```python
from build123d import *

# Parameters (mm, degrees)
SKETCH1_W             = 245.11
SKETCH1_H             = 93.653112922
BOSS_EXTRUDE1_DEPTH   = 2.8575
CUT_EXTRUDE1_REACH    = 4.857
SKETCH2_W             = 181.61
SKETCH2_H             = 3.399764473
CUT_EXTRUDE3_REACH    = 4.857
SKETCH4_W             = 4.572
SKETCH4_H             = 11.676791988
SKETCH4_H_2           = 25.4
CHAMFER2_SIZE         = 0.762
CHAMFER2_SIZE2        = 1.319822715
CHAMFER2_PART_2_SIZE  = 0.762
CHAMFER2_PART_2_SIZE2 = 1.319822715
CHAMFER2_PART_3_SIZE  = 0.762
CHAMFER2_PART_3_SIZE2 = 1.319822715
CHAMFER3_SIZE         = 0.762
CHAMFER3_SIZE2        = 1.319822715
CHAMFER3_PART_2_SIZE  = 0.762
CHAMFER3_PART_2_SIZE2 = 1.319822715
CHAMFER3_PART_3_SIZE  = 0.762
CHAMFER3_PART_3_SIZE2 = 1.319822715
SKETCH6_W             = 11.684
SKETCH6_H             = 0.762
CUT_EXTRUDE4_DEPTH    = 3.8575
SKETCH9_W             = 2.86258
SKETCH9_H             = 12.192
CUT_EXTRUDE5_DEPTH    = 3.8575
SKETCH11_R            = 2.975
CUT_EXTRUDE6_DEPTH    = 3.8575


with BuildPart() as part:
    # Sketch1 → Boss-Extrude1 (new body)
    with BuildSketch(Plane(origin=(0, 0, 0), x_dir=(1, 0, 0), z_dir=(0, 1, 0))):
        Rectangle(SKETCH1_W, SKETCH1_H)
    extrude(amount=BOSS_EXTRUDE1_DEPTH)

    # Sketch2 → Cut-Extrude1 (cut, up to next)
    with BuildSketch(Plane(origin=(0, 2.8575, 0), x_dir=(1, 0, 0), z_dir=(0, 1, 0)), mode=Mode.PRIVATE) as cut_extrude1_sk1:
        with Locations((31.75, 45.126674225)):
            Rectangle(SKETCH2_W, SKETCH2_H)
    cut_extrude1_tool1 = extrude(cut_extrude1_sk1.sketch, amount=-CUT_EXTRUDE1_REACH, mode=Mode.PRIVATE) & part.part
    add(cut_extrude1_tool1.solids().sort_by_distance((31.75, 2.8575, -45.126674))[0], mode=Mode.SUBTRACT)
    # Sketch2 → Cut-Extrude1 (cut, up to next)
    with BuildSketch(Plane(origin=(0, 2.8575, 0), x_dir=(1, 0, 0), z_dir=(0, 1, 0)), mode=Mode.PRIVATE) as cut_extrude1_sk2:
        with Locations((31.75, -45.126674225)):
            Rectangle(SKETCH2_W, SKETCH2_H)
    cut_extrude1_tool2 = extrude(cut_extrude1_sk2.sketch, amount=-CUT_EXTRUDE1_REACH, mode=Mode.PRIVATE) & part.part
    add(cut_extrude1_tool2.solids().sort_by_distance((31.75, 2.8575, 45.126674))[0], mode=Mode.SUBTRACT)

    # Sketch4 → Cut-Extrude3 (cut, up to next)
    with BuildSketch(Plane(origin=(0, 2.8575, 0), x_dir=(1, 0, 0), z_dir=(0, 1, 0)), mode=Mode.PRIVATE) as cut_extrude3_sk1:
        with Locations((120.269, 37.588395994)):
            Rectangle(SKETCH4_W, SKETCH4_H)
    cut_extrude3_tool1 = extrude(cut_extrude3_sk1.sketch, amount=-CUT_EXTRUDE3_REACH, mode=Mode.PRIVATE) & part.part
    add(cut_extrude3_tool1.solids().sort_by_distance((120.269, 2.8575, -37.588396))[0], mode=Mode.SUBTRACT)
    # Sketch4 → Cut-Extrude3 (cut, up to next)
    with BuildSketch(Plane(origin=(0, 2.8575, 0), x_dir=(1, 0, 0), z_dir=(0, 1, 0)), mode=Mode.PRIVATE) as cut_extrude3_sk2:
        with Locations((120.269, -37.588395994)):
            Rectangle(SKETCH4_W, SKETCH4_H)
    cut_extrude3_tool2 = extrude(cut_extrude3_sk2.sketch, amount=-CUT_EXTRUDE3_REACH, mode=Mode.PRIVATE) & part.part
    add(cut_extrude3_tool2.solids().sort_by_distance((120.269, 2.8575, 37.588396))[0], mode=Mode.SUBTRACT)
    # Sketch4 → Cut-Extrude3 (cut, up to next)
    with BuildSketch(Plane(origin=(0, 2.8575, 0), x_dir=(1, 0, 0), z_dir=(0, 1, 0)), mode=Mode.PRIVATE) as cut_extrude3_sk3:
        with Locations((120.269, 0)):
            Rectangle(SKETCH4_W, SKETCH4_H_2)
    cut_extrude3_tool3 = extrude(cut_extrude3_sk3.sketch, amount=-CUT_EXTRUDE3_REACH, mode=Mode.PRIVATE) & part.part
    add(cut_extrude3_tool3.solids().sort_by_distance((120.269, 2.8575, 0))[0], mode=Mode.SUBTRACT)

    # Chamfer2
    chamfer2_edges = [part.edges().sort_by_distance(p)[0] for p in [
        (122.555, 1.42875, 31.75),
    ]]
    chamfer2_side = [part.faces().sort_by_distance(p)[0] for p in [
        (122.555, 1.42875, 22.225),
    ]]
    chamfer(chamfer2_edges, length=CHAMFER2_SIZE, length2=CHAMFER2_SIZE2, reference=chamfer2_side[0])

    # Chamfer2 part 2
    chamfer2_part_2_edges = [part.edges().sort_by_distance(p)[0] for p in [
        (117.983, 1.42875, 43.426791988),
    ]]
    chamfer2_part_2_side = [part.faces().sort_by_distance(p)[0] for p in [
        (117.983, 1.42875, 37.588395994),
    ]]
    chamfer(chamfer2_part_2_edges, length=CHAMFER2_PART_2_SIZE, length2=CHAMFER2_PART_2_SIZE2, reference=chamfer2_part_2_side[0])

    # Chamfer2 part 3
    chamfer2_part_3_edges = [part.edges().sort_by_distance(p)[0] for p in [
        (122.555, 1.42875, -12.7),
    ]]
    chamfer2_part_3_side = [part.faces().sort_by_distance(p)[0] for p in [
        (122.555, 1.42875, -22.225),
    ]]
    chamfer(chamfer2_part_3_edges, length=CHAMFER2_PART_3_SIZE, length2=CHAMFER2_PART_3_SIZE2, reference=chamfer2_part_3_side[0])

    # Chamfer3
    chamfer3_edges = [part.edges().sort_by_distance(p)[0] for p in [
        (122.555, 1.42875, -31.75),
    ]]
    chamfer3_side = [part.faces().sort_by_distance(p)[0] for p in [
        (122.555, 1.42875, -22.606),
    ]]
    chamfer(chamfer3_edges, length=CHAMFER3_SIZE, length2=CHAMFER3_SIZE2, reference=chamfer3_side[0])

    # Chamfer3 part 2
    chamfer3_part_2_edges = [part.edges().sort_by_distance(p)[0] for p in [
        (117.983, 1.42875, -43.426791988),
    ]]
    chamfer3_part_2_side = [part.faces().sort_by_distance(p)[0] for p in [
        (117.983, 1.42875, -37.588395994),
    ]]
    chamfer(chamfer3_part_2_edges, length=CHAMFER3_PART_2_SIZE, length2=CHAMFER3_PART_2_SIZE2, reference=chamfer3_part_2_side[0])

    # Chamfer3 part 3
    chamfer3_part_3_edges = [part.edges().sort_by_distance(p)[0] for p in [
        (122.555, 1.42875, 12.7),
    ]]
    chamfer3_part_3_side = [part.faces().sort_by_distance(p)[0] for p in [
        (122.555, 1.42875, 21.844),
    ]]
    chamfer(chamfer3_part_3_edges, length=CHAMFER3_PART_3_SIZE, length2=CHAMFER3_PART_3_SIZE2, reference=chamfer3_part_3_side[0])

    # Sketch6 → Cut-Extrude4 (cut, through all)
    with BuildSketch(Plane(origin=(0, 2.8575, 0), x_dir=(1, 0, 0), z_dir=(0, 1, 0))):
        with Locations((99.533234068, -0.475391988)):
            Rectangle(SKETCH6_W, SKETCH6_H)
        with Locations((99.533234068, -6.571391988)):
            Rectangle(SKETCH6_W, SKETCH6_H)
        with Locations((99.533234068, -17.802329902)):
            Rectangle(SKETCH6_W, SKETCH6_H)
        with Locations((99.533234068, -23.898329902)):
            Rectangle(SKETCH6_W, SKETCH6_H)
        with Locations((59.401234068, -0.475391988)):
            Rectangle(SKETCH6_W, SKETCH6_H)
        with Locations((59.401234068, -6.571391988)):
            Rectangle(SKETCH6_W, SKETCH6_H)
        with Locations((59.401234068, -17.802329902)):
            Rectangle(SKETCH6_W, SKETCH6_H)
        with Locations((59.401234068, -23.898329902)):
            Rectangle(SKETCH6_W, SKETCH6_H)
        with Locations((19.269234068, -0.475391988)):
            Rectangle(SKETCH6_W, SKETCH6_H)
        with Locations((19.269234068, -6.571391988)):
            Rectangle(SKETCH6_W, SKETCH6_H)
        with Locations((19.269234068, -17.802329902)):
            Rectangle(SKETCH6_W, SKETCH6_H)
        with Locations((19.269234068, -23.898329902)):
            Rectangle(SKETCH6_W, SKETCH6_H)
        with Locations((-20.862765932, -0.475391988)):
            Rectangle(SKETCH6_W, SKETCH6_H)
        with Locations((-20.862765932, -6.571391988)):
            Rectangle(SKETCH6_W, SKETCH6_H)
        with Locations((-20.862765932, -17.802329902)):
            Rectangle(SKETCH6_W, SKETCH6_H)
        with Locations((-20.862765932, -23.898329902)):
            Rectangle(SKETCH6_W, SKETCH6_H)
        with Locations((-60.994765932, -0.475391988)):
            Rectangle(SKETCH6_W, SKETCH6_H)
        with Locations((-60.994765932, -6.571391988)):
            Rectangle(SKETCH6_W, SKETCH6_H)
        with Locations((-60.994765932, -17.802329902)):
            Rectangle(SKETCH6_W, SKETCH6_H)
        with Locations((-60.994765932, -23.898329902)):
            Rectangle(SKETCH6_W, SKETCH6_H)
        with Locations((-101.126765932, -0.475391988)):
            Rectangle(SKETCH6_W, SKETCH6_H)
        with Locations((-101.126765932, -6.571391988)):
            Rectangle(SKETCH6_W, SKETCH6_H)
        with Locations((-101.126765932, -17.802329902)):
            Rectangle(SKETCH6_W, SKETCH6_H)
        with Locations((-101.126765932, -23.898329902)):
            Rectangle(SKETCH6_W, SKETCH6_H)
    extrude(amount=-CUT_EXTRUDE4_DEPTH, mode=Mode.SUBTRACT)

    # Sketch9 → Cut-Extrude5 (cut, through all)
    with BuildSketch(Plane(origin=(0, 2.8575, 0), x_dir=(1, 0, 0), z_dir=(0, 1, 0))):
        with Locations((80.97711923, 0.007208012)):
            Rectangle(SKETCH9_W, SKETCH9_H)
        with Locations((40.84511923, 0.007208012)):
            Rectangle(SKETCH9_W, SKETCH9_H)
        with Locations((40.84511923, -24.376791988)):
            Rectangle(SKETCH9_W, SKETCH9_H)
        with Locations((0.71311923, 0.007208012)):
            Rectangle(SKETCH9_W, SKETCH9_H)
        with Locations((0.71311923, -24.376791988)):
            Rectangle(SKETCH9_W, SKETCH9_H)
        with Locations((80.97711923, -24.376791988)):
            Rectangle(SKETCH9_W, SKETCH9_H)
        with Locations((-39.41888077, 0.007208012)):
            Rectangle(SKETCH9_W, SKETCH9_H)
        with Locations((-39.41888077, -24.376791988)):
            Rectangle(SKETCH9_W, SKETCH9_H)
        with Locations((-79.55088077, 0.007208012)):
            Rectangle(SKETCH9_W, SKETCH9_H)
        with Locations((-79.55088077, -24.376791988)):
            Rectangle(SKETCH9_W, SKETCH9_H)
    extrude(amount=-CUT_EXTRUDE5_DEPTH, mode=Mode.SUBTRACT)

    # Sketch11 → Cut-Extrude6 (cut, through all)
    with BuildSketch(Plane(origin=(0, 2.8575, 0), x_dir=(1, 0, 0), z_dir=(0, 1, 0))):
        with Locations((99.533234068, 13.215208012)):
            Circle(SKETCH11_R)
        with Locations((99.533234068, -37.584791988)):
            Circle(SKETCH11_R)
        with Locations((59.401234068, -37.584791988)):
            Circle(SKETCH11_R)
        with Locations((59.401234068, 13.215208012)):
            Circle(SKETCH11_R)
        with Locations((19.269234068, -37.584791988)):
            Circle(SKETCH11_R)
        with Locations((19.269234068, 13.215208012)):
            Circle(SKETCH11_R)
        with Locations((-20.862765932, -37.584791988)):
            Circle(SKETCH11_R)
        with Locations((-20.862765932, 13.215208012)):
            Circle(SKETCH11_R)
        with Locations((-60.994765932, -37.584791988)):
            Circle(SKETCH11_R)
        with Locations((-60.994765932, 13.215208012)):
            Circle(SKETCH11_R)
        with Locations((-101.126765932, -37.584791988)):
            Circle(SKETCH11_R)
        with Locations((-101.126765932, 13.215208012)):
            Circle(SKETCH11_R)
    extrude(amount=-CUT_EXTRUDE6_DEPTH, mode=Mode.SUBTRACT)


solid = part.part
```
Source: CAD feature listing. Evaluate the final solid. Frame: model axes, mm. Round coordinates to 2 decimals unless told otherwise and drop trailing zeros. Loops run counter-clockwise (first coordinate to the right, second up) from the corner with the lowest first, then second, coordinate; pieces in that order, holes last. Notation, with made-up numbers: M 6,46.25 L 27,46.25 A20 ccw 27,51.25 Z; hole C -6.5,-8.75 d3. An arc over 180 degrees is marked long. Use a Markdown table: item, result. Add a question column.
1. Cut plane C-C, the plane y = 1.1. State how many separate pieces and enclosed holes the cut face has, and give its area (3 significant figures).
2. Cut plane A-A, the plane z = -34. Output: boundary loops of the cut face in (x, y) (1 decimal).
3. Ray query, line 1 along X through (y, z) = (1.8, 23) (3 decimals); line 2 along Z through (x, y) = (-16.5, 0.2); line 3 along X through (y, z) = (0.75, -5.5) (3 decimals). Return the intervals inside material, ascending. Write a range as [from, to].
4. Cut plane B-B, the plane x = 10.5. Output: boundary loops of the cut face in (y, z), and give its area (3 significant figures).
5. Pull-direction query (Z, two-part tool) for faces 1 (the cylindrical face through (-104.1, 1.4, -13.3)), 2 (the flat face through (-2, 2.858, -1)); classes: +Z half, -Z half, draft (parallel to the pull), parting line (faces both ways), or undercut.
6. Contact query for flat-ended pins moving along their axis: pin 1 (0.6 mm diameter, centred on y = 1, z = 0.5, fed in from +X); pin 2 (0.9 mm diameter, centred on x = 81, y = 1, fed in from -Z); pin 3 (4 mm diameter, centred on x = -29, z = 25, fed in from -Y); pin 4 (1.4 mm diameter, centred on x = 19.5, y = 1.5, fed in from +Z). Output: stop coordinate, or through.
Solution:
| question | item | result |
|---|---|---|
| 1 | separate pieces | 1 |
| 1 | enclosed holes | 46 |
| 1 | area | 20,600 mm2 |
| 2 | outline | M -122.6,0 L 118,0 L 118,2.9 L -122.6,2.9 Z |
| 3 | line 1 | x = [-122.555, -80.982], [-78.12, -40.85], [-37.988, -0.718], [2.144, 39.414], [42.276, 79.546], [82.408, 122.555] |
| 3 | line 2 | z = [-43.43, 0.09], [0.86, 6.19], [6.95, 17.42], [18.18, 23.52], [24.28, 43.43] |
| 3 | line 3 | x = [-122.555, -80.982], [-78.12, -40.85], [-37.988, -0.718], [2.144, 39.414], [42.276, 79.546], [82.408, 117.983] |
| 4 | outline | M 0,-43.43 L 2.86,-43.43 L 2.86,43.43 L 0,43.43 Z |
| 4 | area | 248 mm2 |
| 5 | face 1 | undercut |
| 5 | face 2 | draft |
| 6 | pin 1 | stops at x = 117.98 |
| 6 | pin 2 | stops at z = -43.43 |
| 6 | pin 3 | stops at y = 0 |
| 6 | pin 4 | stops at z = 43.43 |
